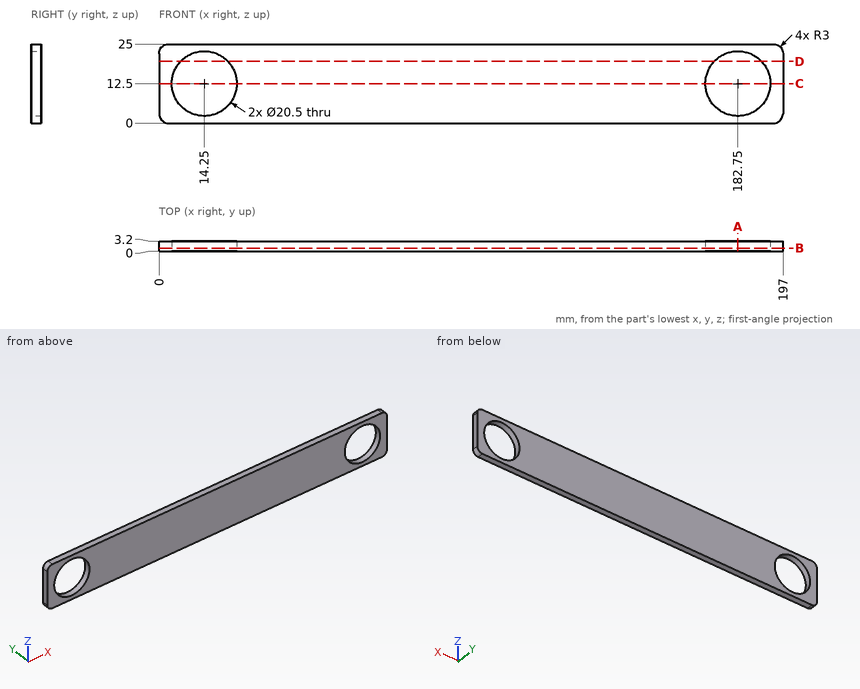
For this review, use the dimensioned drawing (mm, ordinates from the lowest corner) and the shaded views. Coordinates: 2 decimals unless noted, no trailing zeros. Loops run counter-clockwise (first coordinate to the right, second up) from the corner with the lowest first, then second, coordinate; pieces in that order, holes last. Notation, with made-up numbers: (23.25, -12) - (38.25, -12) arc R14 ccw to (38.25, -4) - close; hole circle Ø1 at (-20.75, -3). An arc over 180 degrees is marked (long way). Use CSV: the item, a comma, the result in double quotes. Start each with the question number.
1) For pin 1 Ø12.5 at (x, z) = (14.25, 12.5) entering from -Y (3 decimals), flat-tipped, find the tip position at first contact; note if it passes through.
2) Consider section C-C on z = 12.5. Write out the cut boundary in (x, y), then the cut area to 3 significant figures.
3) Wall thickness on L1, parallel to X at y = 1.65, z = 12.5; L2, parallel to X at y = 3.15, z = 8.5; L3, parallel to Z at x = 19, y = 0.9: over which ranges is each line inside the solid? List them lowest first. Write a range as from..to.
4) Consider section B-B on y = 1. Write out the cut boundary in (x, z).
5) Consider section A-A on x = 182.75. Write out the cut boundary in (y, z), then the cut area to 3 significant figures.
6) Consider section D-D on z = 19.5. Write out the cut boundary in (x, y).
Geometry says:
1,pin 1,"through"
2,outline,"(0, 0) - (4, 0) - (4, 3.2) - (0, 3.2) - close; (24.5, 0) - (172.5, 0) - (172.5, 3.2) - (24.5, 3.2) - close; (193, 0) - (197, 0) - (197, 3.2) - (193, 3.2) - close"
2,area,"499 mm^2"
3,L1,"0..4, 24.5..172.5, 193..197"
3,L2,"0..4.81, 23.69..173.31, 192.19..197"
3,L3,"0..3.42, 21.58..25"
4,outline,"(0, 3) arc R3 ccw to (3, 0) - (194, 0) arc R3 ccw to (197, 3) - (197, 22) arc R3 ccw to (194, 25) - (3, 25) arc R3 ccw to (0, 22) - close; hole circle Ø20.5 at (14.25, 12.5); hole circle Ø20.5 at (182.75, 12.5)"
5,outline,"(0, 0) - (3.2, 0) - (3.2, 2.25) - (0, 2.25) - close; (0, 22.75) - (3.2, 22.75) - (3.2, 25) - (0, 25) - close"
5,area,"14.4 mm^2"
6,outline,"(0, 0) - (6.76, 0) - (6.76, 3.2) - (0, 3.2) - close; (21.74, 0) - (175.26, 0) - (175.26, 3.2) - (21.74, 3.2) - close; (190.24, 0) - (197, 0) - (197, 3.2) - (190.24, 3.2) - close"
